The model under review builds one solid part; all positions refer to its coordinate system, in mm. Round coordinates to 2 decimals unless told otherwise and drop trailing zeros. Order: outer loops, then holes, each group sorted by start corner. A loop starts at its lowest first (then second) coordinate and runs counter-clockwise, first axis right, second up.
```python
from build123d import *

# Parameters (mm, degrees)
SKETCH_R  = 3
PAD_DEPTH = 1.2
FILLET_R  = 0.5


with BuildPart() as part:
    # Sketch → Pad (new body)
    with BuildSketch(Plane.XY):
        with BuildLine():
            ThreePointArc((6, 25), (0, 31), (-6, 25))
            Line((-6, 25), (-6, -25))
            ThreePointArc((-6, -25), (0, -31), (6, -25))
            Line((6, -25), (6, 25))
        make_face()
        with Locations((0, 25)):
            Circle(SKETCH_R, mode=Mode.SUBTRACT)
    extrude(amount=PAD_DEPTH)

    # Fillet
    fillet_edges = [part.edges().sort_by_distance(p)[0] for p in [
        (6, 0, 0),
        (6, 0, 1.2),
    ]]
    fillet(fillet_edges, radius=FILLET_R)


solid = part.part
```
(1) Consider section A-A (x = 0). Write out the cut boundary in (y, z).
Data:
outline: (-31, 0.5) arc R0.5 ccw to (-30.5, 0) - (22, 0) - (22, 1.2) - (-30.5, 1.2) arc R0.5 ccw to (-31, 0.7) - close; (28, 0) - (30.5, 0) arc R0.5 ccw to (31, 0.5) - (31, 0.7) arc R0.5 ccw to (30.5, 1.2) - (28, 1.2) - close
(2) Draft analysis for pull direction X (two halves, no side actions). For faces 1 (the flat face through (0, 0, 1.2)), 2 (the cylindrical face through (-0.65, 22.07, 0.59)), state which applies: pulls with the +X half, pulls with the -X half, needs draft (parallel to the pull), parting line crosses it, or undercut.
Data:
face 1: needs draft
face 2: undercut
(3) To check wall thickness, follow probe 1 along Y at (x, z) = (0, 0.75); probe 2 along Y at (x, z) = (2.75, 0.35); probe 3 along Z at (x, y) = (5.5, -26). State the ranges of each line that lie inside material, in increasing order.
Data:
probe 1: y = -31 to 22, 28 to 31
probe 2: y = -30.31 to 23.8, 26.2 to 30.31
probe 3: z = 0.01 to 1.19
(4) Consider section B-B (z = 0.25). Write out the cut boundary in (x, y), and give its area (3 significant figures).
Data:
outline: (-5.93, -25) arc R5.93 ccw to (5.93, -25) - (5.93, 25) arc R5.93 ccw to (-5.93, 25) - close; hole circle Ø6 at (0, 25)
area: 676 mm2
